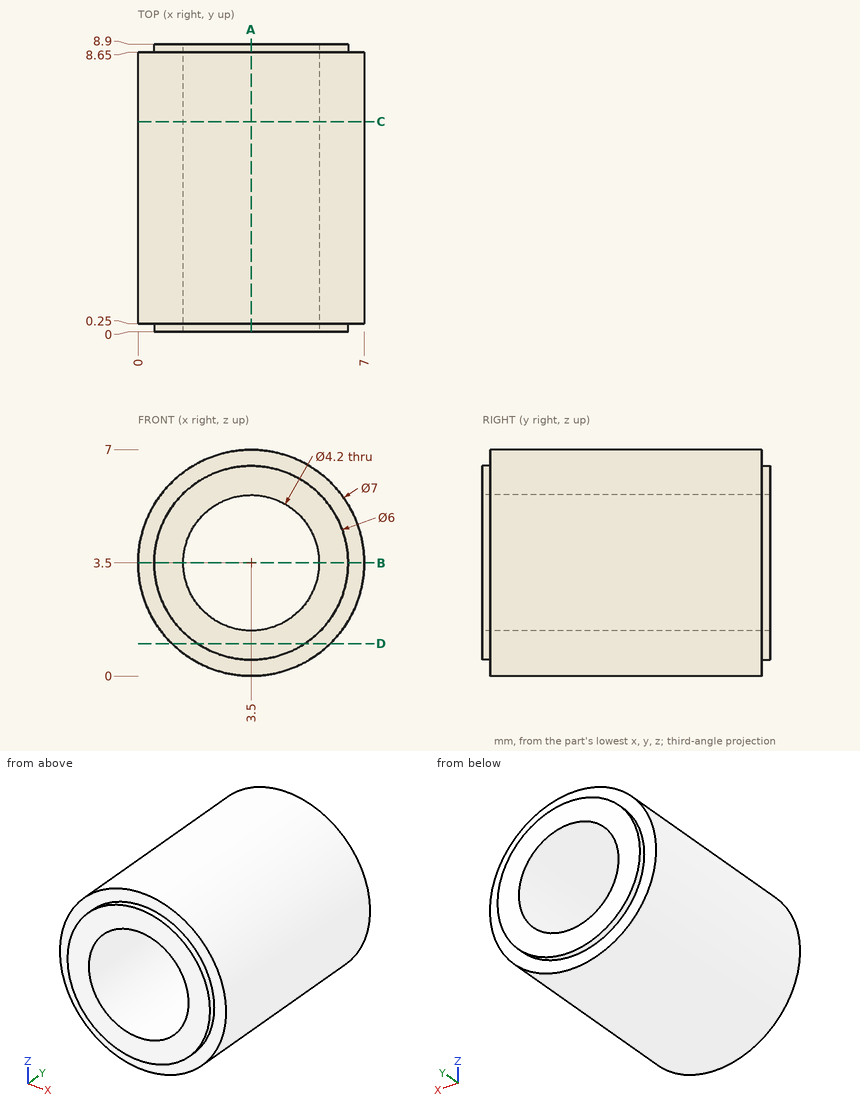
Study the drawing (mm; zero at the part's minimum x, y, z) and answer. Round coordinates to 2 decimals unless told otherwise and drop trailing zeros. Write each loop counter-clockwise with the first axis right and the second up, starting at its lowest first coordinate (ties: lowest second). Pieces come first, ordered by that corner, then holes.
1) A cutting plane is placed at B-B on z = 3.5. Determine the outline of the cut face in (x, y), and give its area (3 significant figures).
2) A cutting plane is placed at C-C on y = 6.5. Determine the outline of the cut face in (x, z).
3) A cutting plane is placed at D-D on z = 1. Determine the outline of the cut face in (x, y), and give its area (3 significant figures).
4) Consider probe 1 along Z at (x, y) = (3.5, 3); probe 2 along Y at (x, z) = (6.25, 5); probe 3 along Z at (x, y) = (2, 8.25). Determine where each line is inside the solid, lowest interval first.
5) A cutting plane is placed at A-A on x = 3.5. Determine the outline of the cut face in (y, z), and give its area (3 significant figures).
6) Flat-ended cylindrical pins translate along their axes: P1, Ø1.5, axis at y = 8, z = 5, coming from the -X side; P2, Ø1.5, axis at y = 7.5, z = 6, coming from the -X side. Find the tip coordinate at first contact, or state that the pin passes through.
Entries:
1. outline: (0, 0.25) - (0.5, 0.25) - (0.5, 0) - (1.4, 0) - (1.4, 8.9) - (0.5, 8.9) - (0.5, 8.65) - (0, 8.65) - close; (5.6, 0) - (6.5, 0) - (6.5, 0.25) - (7, 0.25) - (7, 8.65) - (6.5, 8.65) - (6.5, 8.9) - (5.6, 8.9) - close
1. area: 24.4 mm2
2. outline: circle Ø7 at (3.5, 3.5); hole circle Ø4.2 at (3.5, 3.5)
3. outline: (1.05, 0.25) - (1.84, 0.25) - (1.84, 0) - (5.16, 0) - (5.16, 0.25) - (5.95, 0.25) - (5.95, 8.65) - (5.16, 8.65) - (5.16, 8.9) - (1.84, 8.9) - (1.84, 8.65) - (1.05, 8.65) - close
3. area: 42.8 mm2
4. probe 1: z = 0 to 1.4, 5.6 to 7
4. probe 2: y = 0.25 to 8.65
4. probe 3: z = 0.34 to 2.03, 4.97 to 6.66
5. outline: (0, 0.5) - (0.25, 0.5) - (0.25, 0) - (8.65, 0) - (8.65, 0.5) - (8.9, 0.5) - (8.9, 1.4) - (0, 1.4) - close; (0, 5.6) - (8.9, 5.6) - (8.9, 6.5) - (8.65, 6.5) - (8.65, 7) - (0.25, 7) - (0.25, 6.5) - (0, 6.5) - close
5. area: 24.4 mm2
6. P1: stops at x = 0.08
6. P2: stops at x = 0.47
